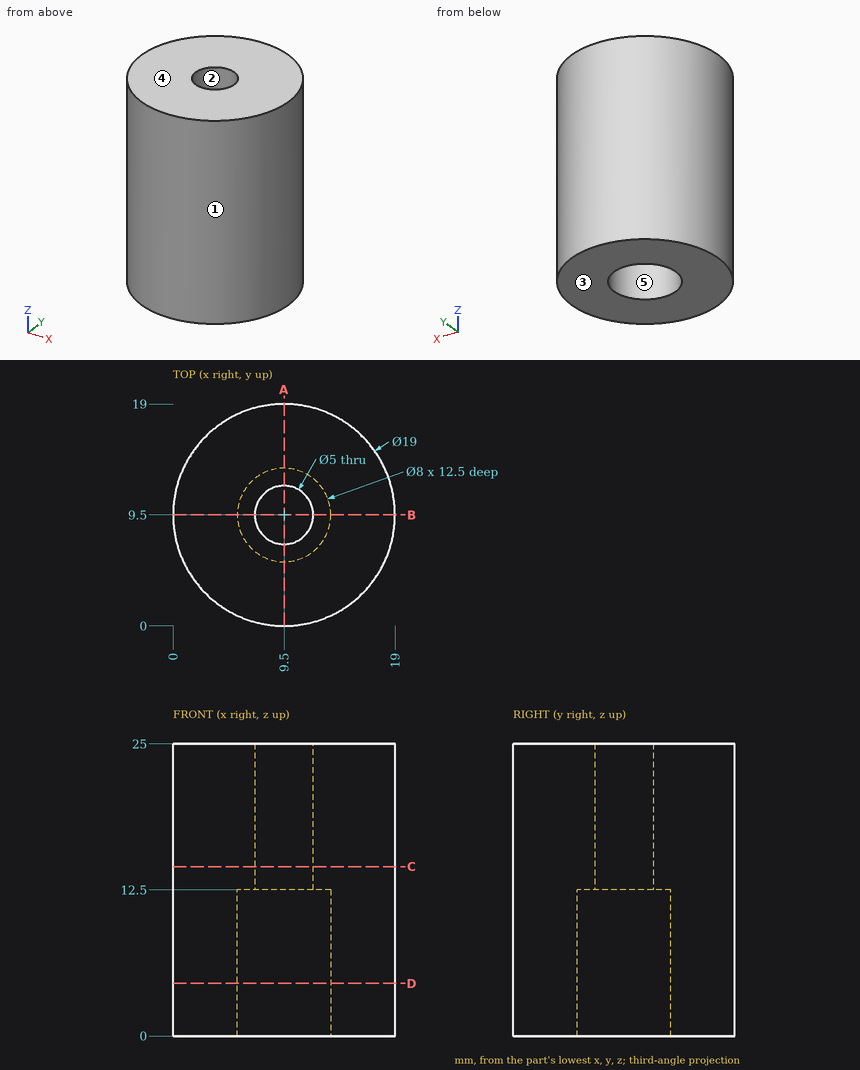
Geometry check sheet. Reference: drawing and pictorial views, mm from the part's lowest x, y, z. A direction names the side the tool comes from. Round coordinates to 2 decimals unless told otherwise and drop trailing zeros. Order: outer loops, then holes, each group sorted by start corner. A loop starts at its lowest first (then second) coordinate and runs counter-clockwise, first axis right, second up. Notation, with made-up numbers: (5.5, -37) - (9.5, -37) arc R24 cw to (9.5, -21) - close; hole circle Ø7 at (76.5, 46.5). An arc over 180 degrees is marked (long way). Use a Markdown table: item, result. Add a question column.
1) Section check A-A (x = 9.5). Record the cut outline in (y, z), then the cut area to 4 significant figures.
2) Section check C-C (z = 14.5). Record the cut outline in (x, y), then the cut area to 3 significant figures.
3) Gauge pin test, flat ends, axial feed: P1, Ø4, axis at x = 15, z = 11, coming from the +Y side; P2, Ø2, axis at y = 4, z = 17.5, coming from the -X side; P3, Ø8, axis at x = 4, y = 10.5, coming from the -Z side; P4, Ø2, axis at x = 12.5, z = 3.5, coming from the -Y side. Record the tip position at first contact, or that the pin passes through.
4) Mould release check, pull along X, two halves, no side actions. Record for the marked faces 1, 2 and 3: released by +X, released by -X, zero draft, split by the parting line, or undercut.
5) Section check D-D (z = 4.5). Record the cut outline in (x, y).
6) Set-up check for the marked faces 4 and 5: record each of +Z, -Z, +X, -X, +Y, -Y from which the full face is reachable in a straight line by a thin tool's end or side.
7) Thickness scan on line 1 along Y through (x, z) = (9.5, 20.5); line 2 along X through (y, z) = (9.25, 4.5); line 3 along Y through (x, z) = (9.5, 3.5). Record the ranges inside material, lowest first.
Established:
| question | item | result |
|---|---|---|
| 1 | outline | (0, 0) - (5.5, 0) - (5.5, 12.5) - (7, 12.5) - (7, 25) - (0, 25) - close; (12, 12.5) - (13.5, 12.5) - (13.5, 0) - (19, 0) - (19, 25) - (12, 25) - close |
| 1 | area | 312.5 mm2 |
| 2 | outline | circle Ø19 at (9.5, 9.5); hole circle Ø5 at (9.5, 9.5) |
| 2 | area | 264 mm2 |
| 3 | P1 | y = 18.33 |
| 3 | P2 | x = 1.13 |
| 3 | P3 | z = 0 |
| 3 | P4 | y = 0.21 |
| 4 | face 1 | split by the parting line |
| 4 | face 2 | undercut |
| 4 | face 3 | zero draft |
| 5 | outline | circle Ø19 at (9.5, 9.5); hole circle Ø8 at (9.5, 9.5) |
| 6 | face 4 | +Z, +X, -X, +Y, -Y |
| 6 | face 5 | -Z |
| 7 | line 1 | 0 to 7, 12 to 19 |
| 7 | line 2 | 0 to 5.51, 13.49 to 19 |
| 7 | line 3 | 0 to 5.5, 13.5 to 19 |
